Part print with two shaded views. Sizes in mm from the minimum x, y, z corner. A direction names the side the tool comes from. Coordinates: 2 decimals unless noted, no trailing zeros. Write each loop counter-clockwise with the first axis right and the second up, starting at its lowest first coordinate (ties: lowest second). Pieces come first, ordered by that corner, then holes. Notation, with made-up numbers: (50, 73.25) -> (108, 73.25) arc R20 cw to (108, 103.25) -> close; hole circle Ø9 at (85.25, 23.5). An arc over 180 degrees is marked (long way). Write item = value, one per line. Start each with the question number.
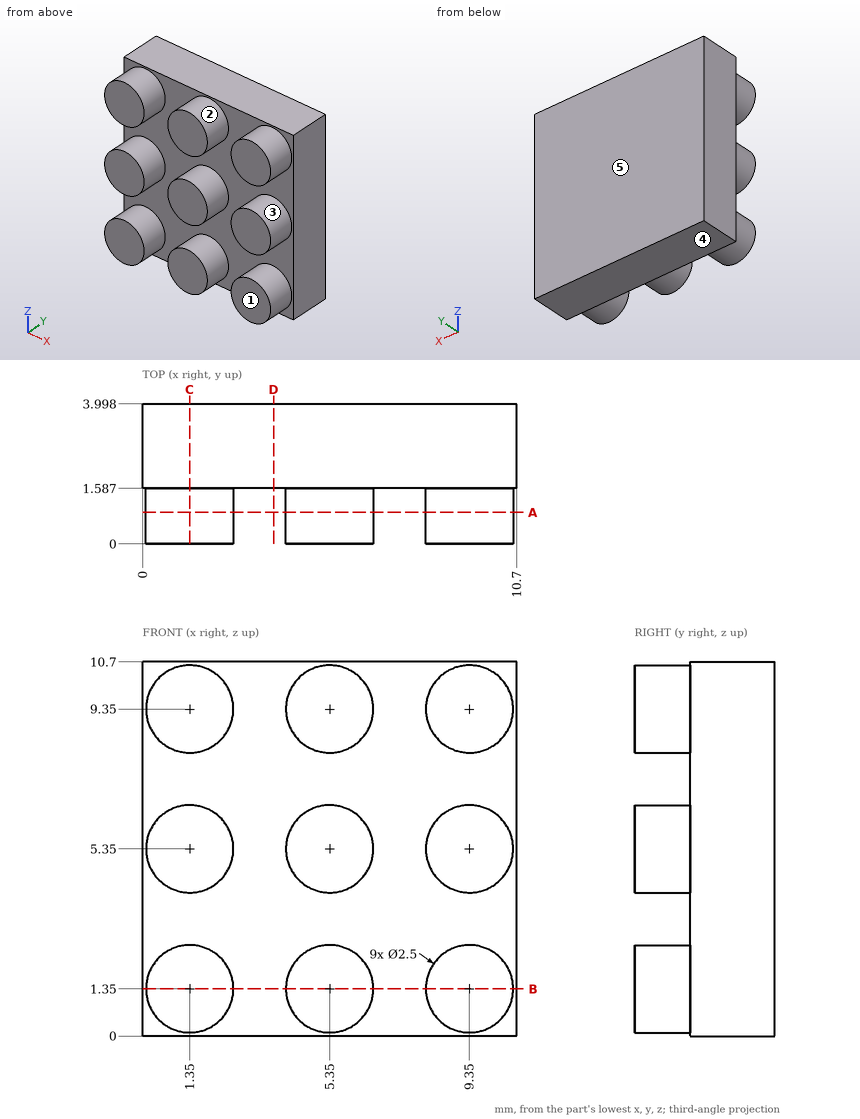
(1) Drop flat-ended pins along their axis: pin 1 Ø5 at (x, z) = (9.5, 7) entering from -Y; pin 2 Ø1 at (x, z) = (3.5, 2) entering from -Y. Give the stop position or say it passes through.
(2) Saw through at C-C (x = 1.35). Give the cut face in (y, z), then the cut area to 3 significant figures.
(3) Drill centre lines: line 1 along X through (y, z) = (1.55, 10); line 2 along X through (y, z) = (1.45, 9.75) (1 decimal); line 3 along Z through (x, y) = (1, 0.8). Where is each one in solid material? Low to high.
(4) Mould opens along Z. For the marked faces 3, 4 and 5 say: released by +Z, released by -Z, zero draft, split by the parting line, or undercut.
(5) Saw through at D-D (x = 3.75). Give the cut face in (y, z).
(6) Saw through at B-B (z = 1.35). Give the cut face in (x, y).
(7) 3-axis set-ups, long thin cutter, end or side, ignore diameter. For the marked faces 1 and 2: which of +Z, -Z, +X, -X, +Y, -Y reach the whole face in a straight line?
(8) Saw through at A-A (y = 0.9). State how many separate pieces and enclosed holes the cut face has.
Returned:
q1.pin_1 = 0
q1.pin_2 = 1.59
q2.outline = (0, 0.1) -> (1.59, 0.1) -> (1.59, 0) -> (4, 0) -> (4, 10.7) -> (1.59, 10.7) -> (1.59, 10.6) -> (0, 10.6) -> (0, 8.1) -> (1.59, 8.1) -> (1.59, 6.6) -> (0, 6.6) -> (0, 4.1) -> (1.59, 4.1) -> (1.59, 2.6) -> (0, 2.6) -> close
q2.area = 37.7 mm2
q3.line_1 = 0.28 to 2.42, 4.28 to 6.42, 8.28 to 10.42
q3.line_2 = 0.2 to 2.5, 4.2 to 6.5, 8.2 to 10.5
q3.line_3 = 0.15 to 2.55, 4.15 to 6.55, 8.15 to 10.55
q4.face_3 = undercut
q4.face_4 = released by -Z
q4.face_5 = zero draft
q5.outline = (1.59, 0) -> (4, 0) -> (4, 10.7) -> (1.59, 10.7) -> close
q6.outline = (0, 1.59) -> (0.1, 1.59) -> (0.1, 0) -> (2.6, 0) -> (2.6, 1.59) -> (4.1, 1.59) -> (4.1, 0) -> (6.6, 0) -> (6.6, 1.59) -> (8.1, 1.59) -> (8.1, 0) -> (10.6, 0) -> (10.6, 1.59) -> (10.7, 1.59) -> (10.7, 4) -> (0, 4) -> close
q7.face_1 = +Z, -Z, +X, -X, -Y
q7.face_2 = -Y
q8.separate_pieces = 9
q8.enclosed_holes = 0
